Part model, mm, in its own coordinate system. Face numbers are marked on the shaded views. A direction names the side the tool comes from. Give positions to 0.01 mm unless a question says otherwise; leave off trailing zeros. Order: outer loops, then holes, each group sorted by start corner. A loop starts at its lowest first (then second) coordinate and runs counter-clockwise, first axis right, second up. Notation, with made-up numbers: (3, 37.25) - (40, 37.25) arc R21 cw to (40, 59.25) - close; hole circle Ø3 at (-35, 61.5). An arc over 180 degrees is marked (long way). Use one line per item in the form item = value. Start each with the question number.
1. Pin check, flat tips, straight feed: P1, Ø1.5, axis at y = 8, z = 32, coming from the -X side; P2, Ø4, axis at y = 13.5, z = 26.5, coming from the -X side; P3, Ø4, axis at y = -8, z = 11.5, coming from the -X side. Stop position of each tip, or through.
2. Drill centre lines: line 1 (Y direction, x = 164.5, z = 6); line 2 (X direction, y = 1, z = 60); line 3 (X direction, y = -8, z = 45.5). Where is each one in solid material? Low to high.
3. Band-saw the part on B-B, the plane x = 173. List the corners of the cut face in (y, z), plus the area to 3 significant figures.
4. Band-saw the part on A-A, the plane y = 0. List the corners of the cut face in (x, z).
5. Band-saw the part on C-C, the plane z = 52.5. List the corners of the cut face in (x, y).
6. Tool access for the marked faces 4 and 5: list every direction of +Z, -Z, +X, -X, +Y, -Y with a clear straight run to the whole face (end or side of a thin tool).
7. Pull direction Y, two halves, no side cores. Call the marked faces 1, 2 and 3: +Y half, -Y half, draft (parallel to the pull), parting line (faces both ways), or undercut.
from build123d import *

# Parameters (mm, degrees)
BOSS_EXTRUDE1_DEPTH = 65
CUT_EXTRUDE1_DEPTH  = 150
BOSS_EXTRUDE2_DEPTH = 65
CUT_EXTRUDE2_DEPTH  = 168
BOSS_EXTRUDE4_DEPTH = 65
CUT_EXTRUDE3_DEPTH  = 225
CUT_EXTRUDE4_DEPTH  = 225


with BuildPart() as part:
    # Sketch1 → Boss-Extrude1 (new body)
    with BuildSketch(Plane.XY):
        with BuildLine():
            Line((0, 18), (470, 18))
            ThreePointArc((470, 18), (488, 0), (470, -18))
            Line((470, -18), (0, -18))
            ThreePointArc((0, -18), (-18, 0), (0, 18))
        make_face()
    extrude(amount=BOSS_EXTRUDE1_DEPTH)

    # Sketch2 → Cut-Extrude1 (cut)
    with BuildSketch(Plane.XY.offset(65)):
        with BuildLine():
            Line((0, -16), (470, -16))
            ThreePointArc((470, -16), (486, 0), (470, 16))
            Line((470, 16), (0, 16))
            ThreePointArc((0, 16), (-16, 0), (0, -16))
        make_face()
    extrude(amount=-CUT_EXTRUDE1_DEPTH, mode=Mode.SUBTRACT)

    # Sketch3 → Boss-Extrude2 (add)
    with BuildSketch(Plane.XY.offset(65)):
        with BuildLine():
            Line((0, -20), (470, -20))
            ThreePointArc((470, -20), (490, 0), (470, 20))
            Line((470, 20), (0, 20))
            ThreePointArc((0, 20), (-20, 0), (0, -20))
        make_face()
    extrude(amount=-BOSS_EXTRUDE2_DEPTH)

    # Sketch4 → Cut-Extrude2 (cut)
    with BuildSketch(Plane.XY.offset(65)):
        with BuildLine():
            Line((0, -18), (470, -18))
            ThreePointArc((470, -18), (488, 0), (470, 18))
            Line((470, 18), (0, 18))
            ThreePointArc((0, 18), (-18, 0), (0, -18))
        make_face()
    extrude(amount=-CUT_EXTRUDE2_DEPTH, mode=Mode.SUBTRACT)

    # Sketch5 → Boss-Extrude4 (add)
    with BuildSketch(Plane.XY.offset(65)):
        with BuildLine():
            Line((0, -18), (470, -18))
            ThreePointArc((470, -18), (488, 0), (470, 18))
            Line((470, 18), (0, 18))
            ThreePointArc((0, 18), (-18, 0), (0, -18))
        make_face()
    extrude(amount=-BOSS_EXTRUDE4_DEPTH)

    # Sketch7 → Cut-Extrude3 (cut)
    with BuildSketch(Plane.XY.offset(65)):
        with BuildLine():
            Line((0, -17), (470, -17))
            ThreePointArc((470, -17), (487, 0), (470, 17))
            Line((470, 17), (0, 17))
            ThreePointArc((0, 17), (-17, 0), (0, -17))
        make_face()
    extrude(amount=-CUT_EXTRUDE3_DEPTH, mode=Mode.SUBTRACT)

    # Sketch8 → Cut-Extrude4 (cut)
    with BuildSketch(Plane.XY.offset(65)):
        with BuildLine():
            Line((0, 20), (470, 20))
            ThreePointArc((470, 20), (490, 0), (470, -20))
            Line((470, -20), (0, -20))
            ThreePointArc((0, -20), (-20, 0), (0, 20))
        make_face()
        with BuildLine():
            Line((0, 19), (470, 19))
            ThreePointArc((470, 19), (489, 0), (470, -19))
            Line((470, -19), (0, -19))
            ThreePointArc((0, -19), (-19, 0), (0, 19))
        make_face(mode=Mode.SUBTRACT)
    extrude(amount=-CUT_EXTRUDE4_DEPTH, mode=Mode.SUBTRACT)


solid = part.part
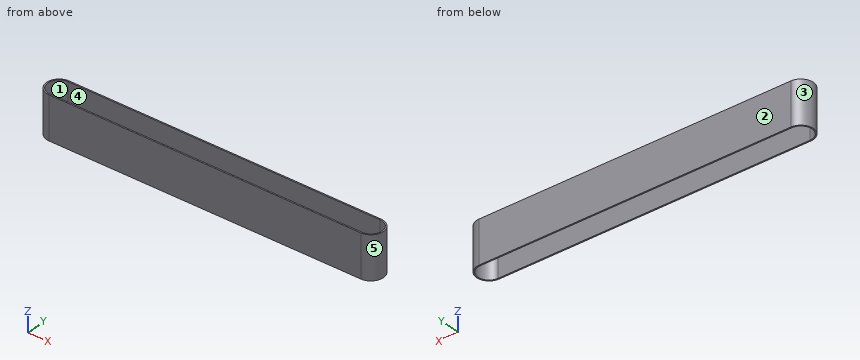
From the geometry:
q1.P1 = -17.56
q1.P2 = -15.12
q1.P3 = -18.03
q2.line_1 = -19 to -17, 17 to 19
q2.line_2 = -18.97 to -16.97, 486.97 to 488.97
q2.line_3 = -17.23 to -15, 485 to 487.23
q3.outline = (-19, 0) - (-17, 0) - (-17, 65) - (-19, 65) - close; (17, 0) - (19, 0) - (19, 65) - (17, 65) - close
q3.area = 260 mm²
q4.outline = (-19, 0) - (-17, 0) - (-17, 65) - (-19, 65) - close; (487, 0) - (489, 0) - (489, 65) - (487, 65) - close
q5.outline = (0, -19) - (470, -19) arc R19 ccw to (470, 19) - (0, 19) arc R19 ccw to start; hole (0, -17) - (470, -17) arc R17 ccw to (470, 17) - (0, 17) arc R17 ccw to start
q6.face_4 = +Z, -Z
q6.face_5 = +Z, -Z, +X
q7.face_1 = undercut
q7.face_2 = +Y half
q7.face_3 = parting line
